```python
from build123d import *

# Parameters (mm, degrees)
PAD_DEPTH       = 20
PAD001_DEPTH    = 20
PAD002_DEPTH    = 20
POCKET_DEPTH    = 5
POCKET001_DEPTH = 40.001
POCKET002_DEPTH = 61.885198
POCKET003_DEPTH = 70.128117


with BuildPart() as part:
    # Sketch → Pad (new body)
    with BuildSketch(Plane.XY):
        Polygon((-17.796612, 26.271189), (12.711864, 30.508476), (36.652542, 11.016947), (36.652542, -22.245762), (12.288136, -41.31356), (-25.423729, -29.661018), (-33.474575, 1.906782), align=None)
    extrude(amount=PAD_DEPTH)

    # Sketch001 (on Face9 of Pad) → Pad001 (join)
    with BuildSketch(Plane.XY.offset(20)):
        Polygon((-8.474573, -15.466103), (-15.677964, -2.966103), (-9.957623, 13.771189), (12.499998, 12.923729), (24.788139, -4.237288), (7.415263, -23.94068), align=None)
    extrude(amount=PAD001_DEPTH)

    # Sketch002 (on Face16 of Pad001) → Pad002 (join)
    with BuildSketch(Plane.XY.offset(40)):
        Polygon((4.872886, -13.347459), (-9.957623, -6.355932), (-9.533896, 3.389829), (3.389833, 9.11017), (13.983051, 3.389829), (15.889828, -5.508473), align=None)
    extrude(amount=PAD002_DEPTH)

    # Sketch003 (on Face16 of Pad002) → Pocket (cut)
    with BuildSketch(Plane.XY.offset(40)):
        Polygon((4.57688, -20.765705), (0, -16.579855), (10.390564, -12.394002), (10.971933, -16.463581), align=None)
    extrude(amount=-POCKET_DEPTH, mode=Mode.SUBTRACT)

    # Sketch004 (on Face16 of Pocket) → Pocket001 (cut, through all)
    with BuildSketch(Plane.XY.offset(40)):
        Polygon((17.64828, -6.177723), (14.857347, 3.009472), (22.888026, -3.350244), (16.187607, -11.682368), align=None)
    extrude(amount=-POCKET001_DEPTH, mode=Mode.SUBTRACT)

    # Sketch005 (on Face28 of Pocket001) → Pocket002 (cut, through all)
    with BuildSketch(Plane(origin=(4.574148, 8.47064, 0), x_dir=(-0.879905, 0.475149, 0), z_dir=(0.475149, 0.879905, 0))):
        Polygon((-8.814835, 53.992447), (-7.755517, 44.67041), (-1.399587, 44.034817), (-2.458905, 53.992447), align=None)
    extrude(amount=-POCKET002_DEPTH, mode=Mode.SUBTRACT)

    # Sketch006 (on Face7 of Pocket002) → Pocket003 (cut, through all)
    with BuildSketch(Plane.YZ.offset(36.652542)):
        Polygon((-11.636175, 6.603847), (-12.483627, 14.019101), (2.346878, 13.171643), (1.28756, 4.908932), align=None)
    extrude(amount=-POCKET003_DEPTH, mode=Mode.SUBTRACT)


solid = part.part
```
Check sheet for the modelled part. Datum: model origin and axes. Units: mm. A direction names the side the tool comes from. Give positions to 0.01 mm unless a question says otherwise; leave off trailing zeros. Write each loop counter-clockwise with the first axis right and the second up, starting at its lowest first coordinate (ties: lowest second). Pieces come first, ordered by that corner, then holes.
Item 1: Gauge pin test, flat ends, axial feed: pin 1 (1.5 mm diameter, centred on x = -14.5, z = 10, fed in from -Y); pin 2 (3 mm diameter, centred on x = 16.5, y = -32, fed in from +Z); pin 3 (4 mm diameter, centred on x = 16, y = -8.5, fed in from +Z). Record the tip position at first contact, or that the pin passes through.
Item 2: Draft check along Y on faces 1 (the face through (-9.75, -1.55, 49.86)), 2 (the face through (3, -2, 60)), 3 (the face through (-28.5, -17.6, 9.9)), 4 (the face through (5, -3, 53.992)). Enter one of: released by +Y, released by -Y, zero draft, split by the parting line, or undercut.
Item 3: Cross-section at A-A (z = 15.5). Enter the section's corners in (x, y).
Item 4: Cross-section at D-D (z = 34). Enter the section's corners in (x, y).
Item 5: Cross-section at C-C (x = 26). Enter the section's corners in (y, z).
Item 6: Cross-section at B-B (y = -2). Enter the section's corners in (x, z), and give its area (3 significant figures).
Item 7: Scan lines: L1, parallel to Z at x = 16, y = -25; L2, parallel to X at y = -23.5, z = 30.5; L3, parallel to Z at x = -20, y = -9.5. Record each from-to range of solid material in increasing order.
Item 8: Access from +Z, -Z, +X, -X, +Y, -Y to the whole of each face (thin tool, end or side, straight path). Record for faces 5 (the face through (7, -17, 35)), 6 (the face through (-3.16, 6.21, 49.86)), 7 (the face through (7.37, -3.804, 49.397)), 8 (the face through (6.26, 7.56, 52.08)).
Report:
1. pin 1: stops at y = -33.27
1. pin 2: stops at z = 20
1. pin 3: stops at z = 40
2. face 1: released by +Y
2. face 2: zero draft
2. face 3: released by -Y
2. face 4: undercut
3. outline: (-33.47, 1.91) - (-25.42, -29.66) - (12.29, -41.31) - (36.65, -22.25) - (36.65, 11.02) - (12.71, 30.51) - (-17.8, 26.27) - close; hole (14.86, 3.01) - (17.65, -6.18) - (16.19, -11.68) - (22.89, -3.35) - close
4. outline: (-15.68, -2.97) - (-8.47, -15.47) - (7.42, -23.94) - (24.79, -4.24) - (12.5, 12.92) - (-9.96, 13.77) - close; hole (14.86, 3.01) - (17.65, -6.18) - (16.19, -11.68) - (22.89, -3.35) - close
5. outline: (-30.58, 0) - (19.69, 0) - (19.69, 20) - (-30.58, 20) - close; hole (-12.48, 14.02) - (-11.64, 6.6) - (1.29, 4.91) - (2.35, 13.17) - close
6. outline: (-32.48, 0) - (16.38, 0) - (16.38, 5.34) - (-32.48, 5.34) - close; (-32.48, 13.42) - (16.38, 13.42) - (16.38, 40) - (15.14, 40) - (15.14, 60) - (-9.77, 60) - (-9.77, 40) - (-15.35, 40) - (-15.35, 20) - (-32.48, 20) - close; (21.18, 0) - (36.65, 0) - (36.65, 5.34) - (21.18, 5.34) - close; (21.18, 13.42) - (36.65, 13.42) - (36.65, 20) - (23.19, 20) - (23.19, 40) - (21.18, 40) - close; hole (0.51, 44.03) - (7.73, 44.67) - (8.94, 53.99) - (1.71, 53.99) - close
6. area: 1,870 mm2
7. L1: z = 0 to 20
7. L2: x = 6.59 to 7.8
7. L3: z = 0 to 6.32, 13.85 to 20
8. face 5: +Z
8. face 6: +Z, -X, +Y
8. face 7: none
8. face 8: +Z, +X, +Y
